Can you work these out from the model? Positions are in its coordinate system, mm. Face numbers are marked on the shaded views. A direction names the side the tool comes from. Give positions to 0.01 mm unless a question says otherwise; leave off trailing zeros. Write each loop counter-clockwise with the first axis right and the second up, starting at its lowest first coordinate (ties: lowest second). Pieces come first, ordered by that corner, then holes. Notation, with made-up numbers: M 25.5,-5 L 45.5,-5 A18 ccw 45.5,20 Z; hole C 43.5,87.5 d8. An arc over 180 degrees is marked long. Answer as CSV lines item,"result". Start each with the question number.
```python
from build123d import *

# Parameters (mm, degrees)
SKETCH1_R           = 25
BOSS_EXTRUDE1_DEPTH = 10
FILLET1_R           = 2
FILLET2_R           = 2
FILLET3_R           = 5
CUT_EXTRUDE2_START  = 26
SKETCH4_W           = 11
SKETCH4_H           = 11
CUT_EXTRUDE2_DEPTH  = 2.5
CIRPATTERN1_COUNT   = 10
SKETCH2_R           = 3.5
CUT_EXTRUDE1_DEPTH  = 21


with BuildPart() as part:
    # Sketch1 → Boss-Extrude1 (new body, symmetric)
    with BuildSketch(Plane.XY):
        Circle(SKETCH1_R)
        with BuildLine():
            Line((-2.01454878, 21.907569313), (-2.01454878, 2.772788518))
            Line((-2.01454878, 2.772788518), (-20.212806743, 8.685760967))
            ThreePointArc((-20.212806743, 8.685760967), (-12.93127555, 17.798373876), (-2.01454878, 21.907569313))
        make_face(mode=Mode.SUBTRACT)
        with BuildLine():
            Line((2.01454878, 21.907569313), (2.01454878, 2.772788518))
            Line((2.01454878, 2.772788518), (20.212806743, 8.685760967))
            ThreePointArc((20.212806743, 8.685760967), (12.93127555, 17.798373876), (2.01454878, 21.907569313))
        make_face(mode=Mode.SUBTRACT)
        with BuildLine():
            Line((21.45786636, 4.853861479), (3.259608397, -1.05911097))
            Line((3.259608397, -1.05911097), (14.506750355, -16.539473817))
            ThreePointArc((14.506750355, -16.539473817), (20.923243358, -6.798373876), (21.45786636, 4.853861479))
        make_face(mode=Mode.SUBTRACT)
        with BuildLine():
            Line((11.247141957, -18.907717943), (0, -3.427355096))
            Line((0, -3.427355096), (-11.247141957, -18.907717943))
            ThreePointArc((-11.247141957, -18.907717943), (0, -22), (11.247141957, -18.907717943))
        make_face(mode=Mode.SUBTRACT)
        with BuildLine():
            Line((-14.506750355, -16.539473817), (-3.259608397, -1.05911097))
            Line((-3.259608397, -1.05911097), (-21.45786636, 4.853861479))
            ThreePointArc((-21.45786636, 4.853861479), (-20.923243358, -6.798373876), (-14.506750355, -16.539473817))
        make_face(mode=Mode.SUBTRACT)
    extrude(amount=BOSS_EXTRUDE1_DEPTH, both=True)

    # Fillet1
    fillet1_edges = [part.edges().sort_by_distance(p)[0] for p in [
        (-25, 0, -10),
        (-25, 0, 10),
    ]]
    fillet(fillet1_edges, radius=FILLET1_R)

    # Fillet2
    fillet2_edges = [part.edges().sort_by_distance(p)[0] for p in [
        (-20.212806743, 8.685760967, 0),
        (-2.01454878, 21.907569313, 0),
        (-14.506750355, -16.539473817, 0),
        (-21.45786636, 4.853861479, 0),
        (11.247141957, -18.907717943, 0),
        (-11.247141957, -18.907717943, 0),
        (21.45786636, 4.853861479, 0),
        (14.506750355, -16.539473817, 0),
        (2.01454878, 21.907569313, 0),
        (20.212806743, 8.685760967, 0),
    ]]
    fillet(fillet2_edges, radius=FILLET2_R)

    # Fillet3
    fillet3_edges = [part.edges().sort_by_distance(p)[0] for p in [
        (-2.01454878, 2.772788518, 0),
        (-3.259608397, -1.05911097, 0),
        (0, -3.427355096, 0),
        (3.259608397, -1.05911097, 0),
        (2.01454878, 2.772788518, 0),
    ]]
    fillet(fillet3_edges, radius=FILLET3_R)

    # Sketch4 → Cut-Extrude2 (cut)
    with BuildSketch(Plane(origin=(0, 0, 0), x_dir=(1, 0, 0), z_dir=(0, 1, 0)).offset(CUT_EXTRUDE2_START)):
        Rectangle(SKETCH4_W, SKETCH4_H)
    cut_extrude2 = extrude(amount=-CUT_EXTRUDE2_DEPTH, mode=Mode.SUBTRACT)

    # CirPattern1: Cut-Extrude2 ×10 about axis
    cirpattern1_axis = Axis((0, 0, 0), (0, 0, 1))
    for i in range(1, CIRPATTERN1_COUNT):
        add(cut_extrude2.rotate(cirpattern1_axis, i * 360 / CIRPATTERN1_COUNT), mode=Mode.SUBTRACT)

    # Sketch2 → Cut-Extrude1 (cut, through all)
    with BuildSketch(Plane(origin=(0, 0, -10), x_dir=(-1, 0, 0), z_dir=(0, 0, -1))):
        Circle(SKETCH2_R)
    extrude(amount=-CUT_EXTRUDE1_DEPTH, mode=Mode.SUBTRACT)


solid = part.part
```
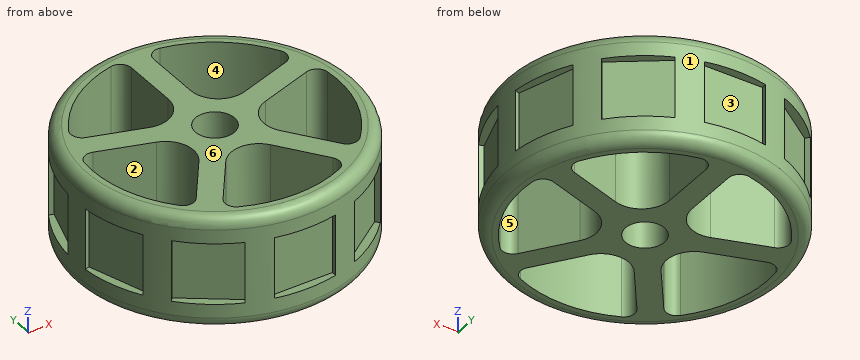
1) On a 3-axis mill with a long thin cutter (end or side, diameter ignored), from which of +Z, -Z, +X, -X, +Y, -Y can I reach the whole of each face in a straight line? I mean the marked faces 5 and 6. Say none if no direction works.
2) I want a section at A-A, the plane x = 0. Please give me the cut outline in (y, z).
3) I need wall thicknesses on L1, parallel to Y at x = 0, z = 5.25; L2, parallel to Y at x = -8, z = -6.25; L3, parallel to Y at x = -3, z = 8.75. Which ranges of each line are inside material? Lowest first, please. Write a range as from..to.
4) I want a section at B-B, the plane z = -3.5. State how many separate pieces and enclosed holes the cut face has, then the cut area to 3 significant figures.
5) Thinking about a two-plate mould opening in Y: for the marked faces 1, 2, 3 and 4, which applies, released by +Y, released by -Y, zero draft, split by the parting line, or undercut?
6) I'm going to push flat-ended pins straight in: P1, Ø3, axis at x = 13, z = -5, coming from the +Y side; P2, Ø4.5, axis at x = 23.5, y = 7.5, coming from the +Z side; P3, Ø1, axis at y = -1.5, z = -5.5, coming from the -X side; P4, Ø2, axis at x = -23.5, y = 6.5, coming from the -Z side. Where does each tip first touch, or does it pass through?
Values found:
1,face 5,"+Z, -Z"
1,face 6,"+Z, +X, -X, +Y, -Y"
2,outline,"M -25,-8 A2 ccw -23,-10 L -22,-10 L -22,10 L -23,10 A2 ccw -25,8 L -25,5.5 L -23.5,5.5 L -23.5,-5.5 L -25,-5.5 Z; M -6.93,-10 L -3.5,-10 L -3.5,10 L -6.93,10 Z; M 3.5,-10 L 23,-10 A2 ccw 25,-8 L 25,-5.5 L 23.5,-5.5 L 23.5,5.5 L 25,5.5 L 25,8 A2 ccw 23,10 L 3.5,10 Z"
3,L1,"y = -23.5..-22, -6.93..-3.5, 3.5..23.5"
3,L2,"y = -23.69..-20.49, -14.44..-7.58, 0.02..4.75, 20.49..23.69"
3,L3,"y = -24.67..-21.79, -7.93..-1.8, 1.8..6.67, 21.32..24.67"
4,separate pieces,"1"
4,enclosed holes,"6"
4,area,"743 mm²"
5,face 1,"split by the parting line"
5,face 2,"undercut"
5,face 3,"released by +Y"
5,face 4,"undercut"
6,P1,"stops at y = 22.15"
6,P2,"stops at z = 10"
6,P3,"stops at x = -24.98"
6,P4,"stops at z = -9.96"
